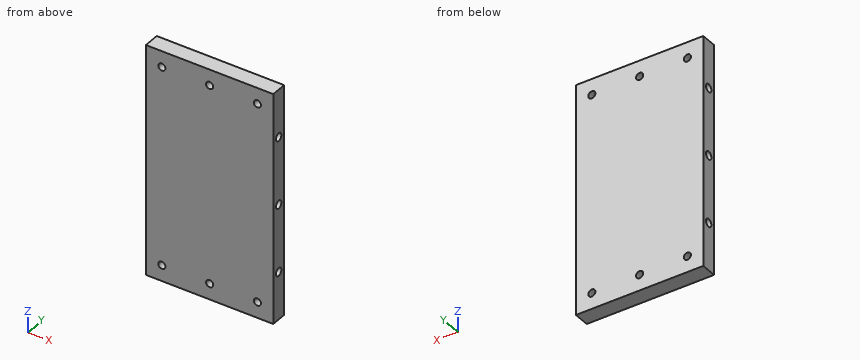
from build123d import *

# Parameters (mm, degrees)
CROQUIS1_W              = 80
CROQUIS1_H              = 145
SALIENTE_EXTRUIR1_DEPTH = 5
CROQUIS2_R              = 2.5
CORTAR_EXTRUIR1_DEPTH   = 10
CROQUIS3_R              = 2.25
CORTAR_EXTRUIR2_DEPTH   = 84.404136588


with BuildPart() as part:
    # Croquis1 → Saliente-Extruir1 (new, symmetric)
    with BuildSketch(Plane(origin=(0, 0, 0), x_dir=(1, 0, 0), z_dir=(0, 1, 0))):
        Rectangle(CROQUIS1_W, CROQUIS1_H)
    extrude(amount=SALIENTE_EXTRUIR1_DEPTH, both=True)

    # Croquis2 → Cortar-Extruir1 (cut)
    with BuildSketch(Plane(origin=(40, 0, 0), x_dir=(0, 0, -1), z_dir=(1, 0, 0))):
        Circle(CROQUIS2_R)
        with Locations((42.5, 0)):
            Circle(CROQUIS2_R)
        with Locations((-42.5, 0)):
            Circle(CROQUIS2_R)
    cortar_extruir1 = extrude(amount=-CORTAR_EXTRUIR1_DEPTH, mode=Mode.SUBTRACT)

    # Simetría1: Cortar-Extruir1 across plane
    add(cortar_extruir1.mirror(Plane(origin=(0, 0, 0), x_dir=(0, 0, 1), z_dir=(1, 0, 0))), mode=Mode.SUBTRACT)

    # Croquis3 → Cortar-Extruir2 (cut, through all)
    with BuildSketch(Plane.XZ.offset(5)):
        with Locations(Location((-30, 62.5, 0), (0, 0, 270))):
            Circle(CROQUIS3_R)
        with Locations(Location((0, 62.5, 0), (0, 0, 270))):
            Circle(CROQUIS3_R)
        with Locations(Location((30, 62.5, 0), (0, 0, 270))):
            Circle(CROQUIS3_R)
        with Locations(Location((30, -62.5, 0), (0, 0, 90))):
            Circle(CROQUIS3_R)
        with Locations(Location((0, -62.5, 0), (0, 0, 90))):
            Circle(CROQUIS3_R)
        with Locations(Location((-30, -62.5, 0), (0, 0, 90))):
            Circle(CROQUIS3_R)
    extrude(amount=-CORTAR_EXTRUIR2_DEPTH, mode=Mode.SUBTRACT)


solid = part.part
Check sheet for the modelled part. Datum: model origin and axes. Units: mm. Give positions to 0.01 mm unless a question says otherwise; leave off trailing zeros. Loops run counter-clockwise (first coordinate to the right, second up) from the corner with the lowest first, then second, coordinate; pieces in that order, holes last. Notation, with made-up numbers: M 15.25,64.5 L 35.25,64.5 A22 ccw 35.25,96.5 Z; hole C 0,80.5 d8. An arc over 180 degrees is marked long. Use a Markdown table: item, result. Add a question column.
Q1. Sectioned sample at A-A, the plane z = -62.5. Record the cut outline in (x, y).
Q2. Go/stop test with flat-tipped pins: pin 1 (3 mm diameter, centred on y = 0, z = -42.5, fed in from +X); pin 2 (1.5 mm diameter, centred on y = 0, z = 41.5, fed in from -X); pin 3 (4 mm diameter, centred on x = -30, z = 62.5, fed in from -Y). Record where each tip stops, or that it passes through.
Q3. Sectioned sample at C-C, the plane z = -42.5. Record the cut outline in (x, y).
Q4. Sectioned sample at B-B, the plane x = 0. Record the cut outline in (y, z), then the cut area to 3 significant figures.
Q5. Scan lines: line 1 along X through (y, z) = (-2, 62.5); line 2 along Y through (x, z) = (-36, 0); line 3 along Y through (x, z) = (37, 42). Record each from-to range of solid material in increasing order. Write a range as [from, to].
Verdict:
| question | item | result |
|---|---|---|
| 1 | outline | M -40,-5 L -32.25,-5 L -32.25,5 L -40,5 Z; M -27.75,-5 L -2.25,-5 L -2.25,5 L -27.75,5 Z; M 2.25,-5 L 27.75,-5 L 27.75,5 L 2.25,5 Z; M 32.25,-5 L 40,-5 L 40,5 L 32.25,5 Z |
| 2 | pin 1 | x = 30 |
| 2 | pin 2 | x = -30 |
| 2 | pin 3 | through |
| 3 | outline | M -40,-5 L 40,-5 L 40,-2.5 L 30,-2.5 L 30,2.5 L 40,2.5 L 40,5 L -40,5 L -40,2.5 L -30,2.5 L -30,-2.5 L -40,-2.5 Z |
| 4 | outline | M -5,-72.5 L 5,-72.5 L 5,-64.75 L -5,-64.75 Z; M -5,-60.25 L 5,-60.25 L 5,60.25 L -5,60.25 Z; M -5,64.75 L 5,64.75 L 5,72.5 L -5,72.5 Z |
| 4 | area | 1,360 mm^2 |
| 5 | line 1 | [-40, -32.25], [-27.75, -2.25], [2.25, 27.75], [32.25, 40] |
| 5 | line 2 | [-5, -2.5], [2.5, 5] |
| 5 | line 3 | [-5, -2.45], [2.45, 5] |
